Input: dimensioned drawing with shaded views. Units: mm. Origin: part minimum x, y, z. A direction names the side the tool comes from. Give positions to 0.01 mm unless a question says otherwise; leave off trailing zeros. Write each loop counter-clockwise with the first axis right and the second up, starting at its lowest first coordinate (ties: lowest second). Pieces come first, ordered by that corner, then holes. Notation, with made-up numbers: M 44.5,-31.5 L 48.5,-31.5 A11 ccw 48.5,-19.5 Z; hole C 4.5,-23.5 d10. An arc over 180 degrees is marked long. Answer as a JSON object with one key per item and string values.
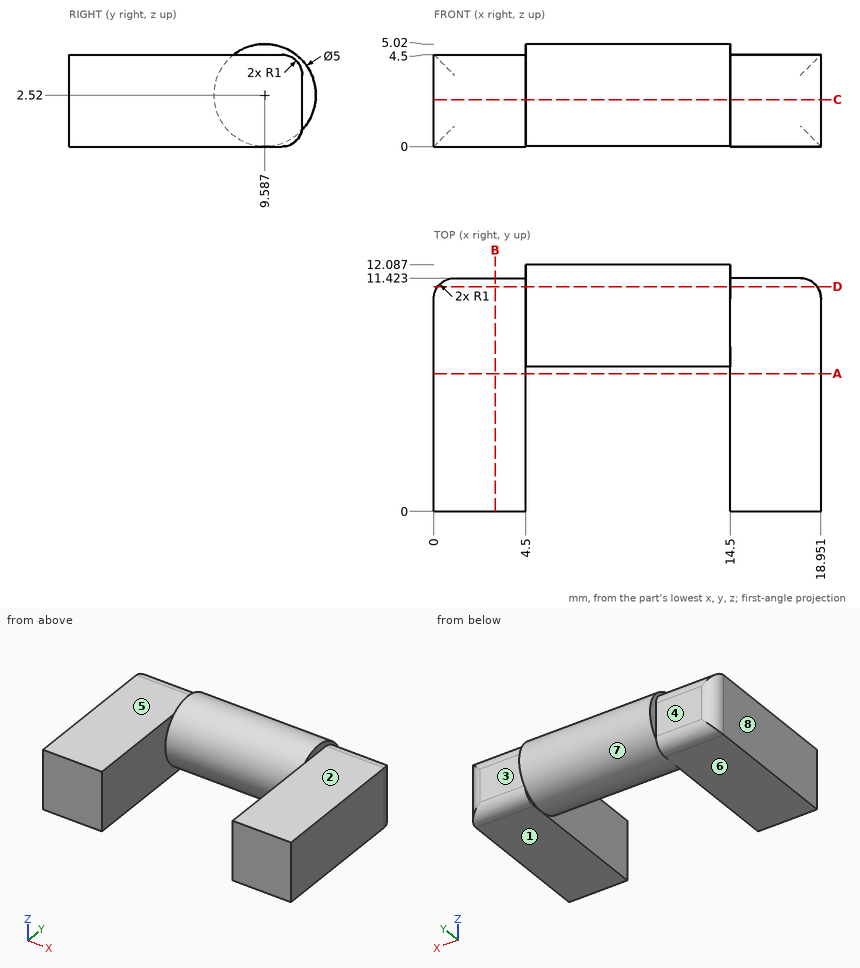
1) Pull-direction query (X, two-part tool) for the marked faces 6, 7 and 8; classes: pulls with the +X half, pulls with the -X half, needs draft (parallel to the pull), parting line crosses it, or undercut.
Geometry check:
{"face 6": "needs draft", "face 7": "undercut", "face 8": "pulls with the -X half"}
2) Cut plane C-C on z = 2.3. Return loops of the section in (x, y), and give its area (3 significant figures).
Geometry check:
{"outline": "M 0,0 L 4.5,0 L 4.5,7.1 L 14.5,7.1 L 14.5,0 L 18.95,0 L 18.95,10.42 A1 ccw 17.95,11.42 L 14.5,11.42 L 14.5,12.08 L 4.5,12.08 L 4.5,11.42 L 1,11.42 A1 ccw 0,10.42 Z", "area": "152 mm2"}
3) Line query: line 1 (X direction, y = 5.5, z = 2.85); line 2 (Y direction, x = 3.75, z = 3.5); line 3 (Z direction, x = 2.25, y = 9.5). Output: solid intervals per line, ascending. Write a range as from..to.
Geometry check:
{"line 1": "x = 0..4.5, 14.5..18.95", "line 2": "y = 0..11.42", "line 3": "z = 0..4.5"}
4) Cut plane D-D on y = 11. Return loops of the section in (x, z).
Geometry check:
{"outline": "M 0.18,0.18 L 4.5,0.18 L 4.5,0.46 L 14.5,0.46 L 14.5,0.18 L 18.77,0.18 L 18.77,4.32 L 14.5,4.32 L 14.5,4.58 L 4.5,4.58 L 4.5,4.32 L 0.18,4.32 Z"}
5) Set-up query: the marked faces 1, 2, 3, 4 and 5. Return all of +Z, -Z, +X, -X, +Y, -Y with unobstructed straight access to the full face (end or side cutting, diameter ignored); none if empty.
Geometry check:
{"face 1": "-Z, +X, -X, +Y, -Y", "face 2": "+Z, +X, +Y, -Y", "face 3": "+Z, -Z, +X, +Y", "face 4": "+Z, -Z, -X, +Y", "face 5": "+Z, -X, +Y, -Y"}
6) Cut plane B-B on x = 3. Return loops of the section in (y, z).
Geometry check:
{"outline": "M 0,0 L 10.42,0 A1 ccw 11.42,1 L 11.42,3.5 A1 ccw 10.42,4.5 L 0,4.5 Z"}
7) Cut plane A-A on y = 6.75. Return loops of the section in (x, z).
Geometry check:
{"outline": "M 0,0 L 4.5,0 L 4.5,4.5 L 0,4.5 Z; M 14.5,0 L 18.95,0 L 18.95,4.5 L 14.5,4.5 Z"}
8) Contact query for flat-ended pins moving along their axis: P1, Ø6, axis at x = 16, y = 4.5, coming from the +Z side; P2, Ø2, axis at x = 3, z = 3, coming from the +Y side; P3, Ø2, axis at x = 11.5, z = 1.5, coming from the -Y side. Output: stop coordinate, or through.
Geometry check:
{"P1": "stops at z = 4.5", "P2": "stops at y = 11.42", "P3": "stops at y = 7.09"}
